Job drawing, mm, ordinate dimensions from the low corner. One solid piece. A direction names the side the tool comes from. Coordinates: 2 decimals unless noted, no trailing zeros. Loops run counter-clockwise (first coordinate to the right, second up) from the corner with the lowest first, then second, coordinate; pieces in that order, holes last. Notation, with made-up numbers: (51.5, 67) -> (70.5, 67) arc R26 ccw to (70.5, 102) -> close; hole circle Ø2 at (66.25, 77.5). An arc over 180 degrees is marked (long way). Use one line per item in the form item = value. Start each with the question number.
(1) Pin check, flat tips, straight feed: P1, Ø2, axis at x = 19, z = 29, coming from the -Y side; P2, Ø2.5, axis at x = 69, z = 24, coming from the +Y side; P3, Ø5.5, axis at x = 60, z = 14, coming from the +Y side; P4, Ø1.6, axis at y = 89, z = 11, coming from the +X side. Stop position of each tip, or through.
(2) Mould opens along Y. For the marked faces 1, 2, 3 and 4 say: +Y half, -Y half, draft (parallel to the pull), parting line (faces both ways), or undercut.
(3) Band-saw the part on B-B on z = 6. Give the cut face in (x, y).
(4) Band-saw the part on D-D on z = 22.5. Give the cut face in (x, y).
(5) 3-axis set-ups, long thin cutter, end or side, ignore diameter. For the marked faces 5 and 6: which of +Z, -Z, +X, -X, +Y, -Y reach the whole face in a straight line?
(6) Band-saw the part on A-A on y = 54. Give the cut face in (x, z), then the cut area to 3 significant figures.
(7) Drill centre lines: L1, parallel to X at y = 58.5, z = 13; L2, parallel to Y at x = 18.5, z = 24; L3, parallel to X at y = 76.25, z = 14. Where is each one in solid material? Low to high. Write a range as [from, to].
(8) Band-saw the part on C-C on z = 14. Give the cut face in (x, y), then the cut area to 3 significant figures.
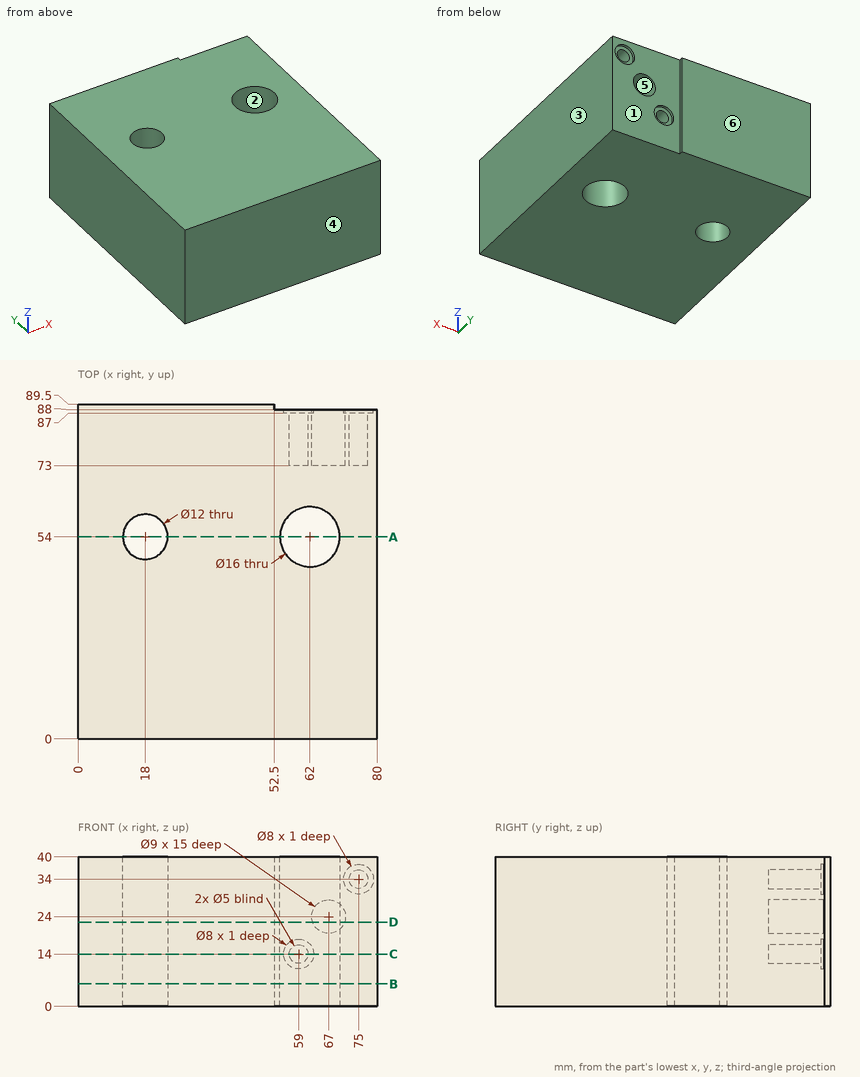
A:
q1.P1 = 0
q1.P2 = 73
q1.P3 = 87
q1.P4 = 52.5
q2.face_1 = +Y half
q2.face_2 = undercut
q2.face_3 = draft
q2.face_4 = -Y half
q3.outline = (0, 0) -> (80, 0) -> (80, 88) -> (52.5, 88) -> (52.5, 89.5) -> (0, 89.5) -> close; hole circle Ø12 at (18, 54); hole circle Ø16 at (62, 54)
q4.outline = (0, 0) -> (80, 0) -> (80, 88) -> (71.24, 88) -> (71.24, 73) -> (62.76, 73) -> (62.76, 88) -> (52.5, 88) -> (52.5, 89.5) -> (0, 89.5) -> close; hole circle Ø12 at (18, 54); hole circle Ø16 at (62, 54)
q5.face_5 = +Y
q5.face_6 = +Z, -Z, +X, -X, +Y
q6.outline = (0, 0) -> (12, 0) -> (12, 40) -> (0, 40) -> close; (24, 0) -> (54, 0) -> (54, 40) -> (24, 40) -> close; (70, 0) -> (80, 0) -> (80, 40) -> (70, 40) -> close
q6.area = 2,080 mm²
q7.L1 = [0, 14.03], [21.97, 55.39], [68.61, 80]
q7.L2 = [0, 48.02], [59.98, 89.5]
q7.L3 = [0, 56.5], [61.5, 80]
q8.outline = (0, 0) -> (80, 0) -> (80, 88) -> (63, 88) -> (63, 87) -> (61.5, 87) -> (61.5, 73) -> (56.5, 73) -> (56.5, 87) -> (55, 87) -> (55, 88) -> (52.5, 88) -> (52.5, 89.5) -> (0, 89.5) -> close; hole circle Ø12 at (18, 54); hole circle Ø16 at (62, 54)
q8.area = 6,730 mm²
